from build123d import *

# Parameters (mm, degrees)
F0_R     = 8
F1_DEPTH = 3
F2_R     = 6
F3_DEPTH = 15
F4_R     = 8
F4_R_2   = 6
F5_DEPTH = 3
F6_R     = 1.49999
F7_W     = 3
F7_H     = 3


# Not quite as in the source:
# - a fillet or chamfer is up to 0.001 mm smaller than in the source, because OpenCascade refuses the exact size


with BuildPart() as f1:
    # F0 (on Top) → F1 (new body)
    with BuildSketch(Plane.XY):
        Circle(F0_R)
    extrude(amount=F1_DEPTH)

    # F2 (on face) → F3 (join)
    with BuildSketch(Plane.XY.offset(3)):
        Circle(F2_R)
    extrude(amount=F3_DEPTH)

    # F4 (on face) → F5 (join)
    with BuildSketch(Plane.XY.offset(18)):
        Circle(F4_R)
        Circle(F4_R_2, mode=Mode.SUBTRACT)
        Circle(F4_R_2)
    extrude(amount=F5_DEPTH)

    # F6 (radius 1.5 in the source; OpenCascade refuses exactly that, so slightly less here)
    f6_edges = [f1.edges().sort_by_distance(p)[0] for p in [
        (-8, 0, 21),
        (-8, 0, 18),
        (-8, 0, 3),
        (-8, 0, 0),
    ]]
    fillet(f6_edges, radius=F6_R)

    # F7 (on Front) → F8 (revolve, cut)
    with BuildSketch(Plane.XZ):
        with Locations((4.5, 4.5)):
            Rectangle(F7_W, F7_H)
        with Locations((4.5, 16.5)):
            Rectangle(F7_W, F7_H)
    revolve(axis=Axis((0, 0, 11.7473863065), (0, 0, 1)), mode=Mode.SUBTRACT)


solid = f1.part
Model file for the job. Use its own axes, mm. Give positions to 0.01 mm unless a question says otherwise; leave off trailing zeros. Write each loop counter-clockwise with the first axis right and the second up, starting at its lowest first coordinate (ties: lowest second). Pieces come first, ordered by that corner, then holes. Notation, with made-up numbers: (36, -22.5) - (76, -22.5) arc R15 cw to (76, -1.5) - close; hole circle Ø10 at (51.25, 54.5). An arc over 180 degrees is marked (long way). Answer as CSV lines item,"result".
1. Drill centre lines: L1, parallel to Z at x = -3.5, y = 1.25; L2, parallel to Z at x = 2.75, y = 5.75; L3, parallel to Z at x = -6.75, y = 3.75. Where is each one in solid material? Low to high. Write a range as [from, to].
Responses:
L1,"z = [0, 3], [6, 15], [18, 21]"
L2,"z = [0, 3], [18, 21]"
L3,"z = [0.63, 2.37], [18.63, 20.37]"
2. Pin check, flat tips, straight feed: pin 1 (2 mm diameter, centred on x = 4, z = 3, fed in from -Y); pin 2 (2 mm diameter, centred on x = 4.5, z = 15.5, fed in from -Y); pin 3 (3 mm diameter, centred on x = 2.5, z = 10, fed in from -Y). Stop position of each tip, or through.
Responses:
pin 1,"stops at y = -7.05"
pin 2,"stops at y = -4.77"
pin 3,"stops at y = -5.92"
3. Band-saw the part on C-C (z = 5.75). Write the cut outline in (x, y), and give its area (3 significant figures).
Responses:
outline,"circle Ø6 at (0, 0)"
area,"28.3 mm2"
4. Band-saw the part on D-D (x = 5). Count the separate pieces of the cut face and the enclosed holes in it, and give its area (3 significant figures).
Responses:
separate pieces,"3"
enclosed holes,"0"
area,"130 mm2"
5. Two-plate mould, pull along Z, no slides. Class faces 1 (the face through (0, 0, 0)), 2 (the face through (-1, -3, 3)), 3 (the face through (0, 0, 21)), 4 (the face through (-6, 0, 10)): +Z half, -Z half, draft (parallel to the pull), parting line (faces both ways), or undercut.
Responses:
face 1,"-Z half"
face 2,"undercut"
face 3,"+Z half"
face 4,"undercut"
